from build123d import *

# Parameters (mm, degrees)
F0_R     = 1.27
F1_DEPTH = 2.54
F2_W     = 2.54
F2_H     = 5.08
F3_DEPTH = 2.54
F4_W     = 2.54
F4_H     = 2.54
F4_R     = 0.680019
F5_DEPTH = 25.4


with BuildPart() as f1:
    # F0 (on Front) → F1 (new body)
    with BuildSketch(Plane.XZ):
        with BuildLine():
            ThreePointArc((-32.792888, 1.933751), (-35.332888, 4.468064), (-37.872888, 1.933751))
            Line((-37.872888, 1.933751), (-37.872888, -20.926249))
            Line((-37.872888, -20.926249), (-32.792888, -20.926249))
            Line((-32.792888, -20.926249), (-32.792888, 1.933751))
        make_face()
        with Locations((-35.332888, 1.933751)):
            Circle(F0_R, mode=Mode.SUBTRACT)
    extrude(amount=F1_DEPTH)

    # F2 (on face) → F3 (join)
    with BuildSketch(Plane(origin=(-37.872888, 0, 0), x_dir=(0, -1, 0), z_dir=(-1, 0, 0))):
        with Locations((1.27, -18.386249)):
            Rectangle(F2_W, F2_H)
    extrude(amount=F3_DEPTH)

    # F4 (on face) → F5 (cut)
    with BuildSketch(Plane.XZ.offset(2.54)):
        with Locations((-39.142888, -17.116249)):
            Rectangle(F4_W, F4_H)
        with Locations((-39.142888, -19.656249)):
            Circle(F4_R)
        with BuildLine():
            ThreePointArc((-39.142888, -20.926249), (-40.040536, -20.553897), (-40.412888, -19.656249))
            Line((-40.412888, -19.656249), (-40.412888, -20.926249))
            Line((-40.412888, -20.926249), (-39.142888, -20.926249))
        make_face()
    extrude(amount=-F5_DEPTH, mode=Mode.SUBTRACT)


solid = f1.part
Design review of the part built by this model. Coordinates are the model's own, in mm. A direction names the side the tool comes from. Coordinates: 2 decimals unless noted, no trailing zeros. Loops run counter-clockwise (first coordinate to the right, second up) from the corner with the lowest first, then second, coordinate; pieces in that order, holes last. Notation, with made-up numbers: (4, 49) - (24, 49) arc R19 ccw to (24, 77) - close; hole circle Ø10 at (-27, 23.25). An arc over 180 degrees is marked (long way). Use CSV: the item, a comma, the result in double quotes. Start each with the question number.
1. Add section C-C on z = -11.25. Give the boundary of the cut face in (x, y).
2. Mouldability with a two-part tool opening along X and no side actions: class faces 3 (the cylindrical face through (-40.031, -1.288, -20.564)), 4 (the flat face through (-36, -1, -20.926)), 5 (the cylindrical face through (-35.277, -1.252, 4.467)), 6 (the cylindrical face through (-36.6, -1.3, 2)) as released by +X, released by -X, zero draft, split by the parting line, or undercut.
3. For faces 1 (the cylindrical face through (-39.644, -1.288, -19.197)), 2 (the flat face through (-37.873, -1, -8)), list the 3-axis set-ups (+Z, -Z, +X, -X, +Y, -Y) from which the entire face can be reached by the end or side of a thin tool; tool diameter is ignored.
4. To check wall thickness, follow probe 1 along Z at (x, y) = (-38.25, -2.3); probe 2 along X at (y, z) = (-1.05, -14); probe 3 along Z at (x, y) = (-39, -0.85). State the ranges of each line that lie inside material, in increasing order.
5. Add section B-B on x = -38.75. Give the boundary of the cut face in (y, z), plus the area to 3 significant figures.
6. Add section A-A on y = -2. Give the boundary of the cut face in (x, z), plus the area to 3 significant figures.
7. Clearance check with flat-ended pins moving along their axes: pin 1 (1.8 mm diameter, centred on x = -39.14, z = -19.66, fed in from -Y); pin 2 (1 mm diameter, centred on x = -39, y = -0.5, fed in from +Z); pin 3 (1.3 mm diameter, centred on y = -1, z = -7, fed in from -X). State where each tip first meets the part, or that it passes through.
8. Add section D-D on x = -36.25. Give the boundary of the cut face in (y, z).
Resolved:
1,outline,"(-37.87, -2.54) - (-32.79, -2.54) - (-32.79, 0) - (-37.87, 0) - close"
2,face 3,"released by -X"
2,face 4,"zero draft"
2,face 5,"split by the parting line"
2,face 6,"undercut"
3,face 1,"+Y, -Y"
3,face 2,"+Z, -X, +Y, -Y"
4,probe 1,"-20.93 to -18.39"
4,probe 2,"-37.87 to -32.79"
4,probe 3,"-20.93 to -20.32, -18.99 to -18.39"
5,outline,"(-2.54, -20.93) - (0, -20.93) - (0, -20.21) - (-2.54, -20.21) - close; (-2.54, -19.1) - (0, -19.1) - (0, -18.39) - (-2.54, -18.39) - close"
5,area,"3.63 mm2"
6,outline,"(-40.41, -19.66) arc R1.27 ccw to (-39.14, -20.93) - (-32.79, -20.93) - (-32.79, 1.93) arc R2.54 ccw to (-37.87, 1.93) - (-37.87, -18.39) - (-40.41, -18.39) - close; hole circle Ø1.36 at (-39.14, -19.66); hole circle Ø2.54 at (-35.33, 1.93)"
6,area,"126 mm2"
7,pin 1,"y = -2.54"
7,pin 2,"z = -18.39"
7,pin 3,"x = -37.87"
8,outline,"(-2.54, -20.93) - (0, -20.93) - (0, 1.06) - (-2.54, 1.06) - close; (-2.54, 2.81) - (0, 2.81) - (0, 4.3) - (-2.54, 4.3) - close"
